Geometry: final body of the model. Coordinates: model frame, mm. A direction names the side the tool comes from. Coordinates: 2 decimals unless noted, no trailing zeros. Write each loop counter-clockwise with the first axis right and the second up, starting at its lowest first coordinate (ties: lowest second). Pieces come first, ordered by that corner, then holes.
from build123d import *

# Parameters (mm, degrees)
F0_W     = 150
F0_H     = 35
F1_DEPTH = 40
F2_D     = 5
F2_DEPTH = 50
F2_TIP   = 1.5021515476
F4_D     = 12
F4_DEPTH = 50
F4_TIP   = 3.6051637142
F5_D     = 20
F5_DEPTH = 50
F5_TIP   = 6.0086061903


with BuildPart() as f1:
    # F0 (on Top) → F1 (new body)
    with BuildSketch(Plane.XY):
        with Locations((0.152673311, -0.1323037595)):
            Rectangle(F0_W, F0_H)
    extrude(amount=F1_DEPTH)

    # F2
    with Locations(Plane(origin=(0, 0, 0), x_dir=(1, 0, 0), z_dir=(0, 0, -1))):
        with Locations((-59, -7.4576994487), (-69, 0.0423005513), (-59, 7.5423005513), (-49, 0.0423005513), (49, 0.0423005513), (59, -7.4576994487), (59, 7.5423005513), (69, 0.0423005513)):
            Hole(F2_D / 2, depth=F2_DEPTH)
            with Locations((0, 0, -(F2_DEPTH + F2_TIP / 2))):  # 118° drill point
                Cone(0, F2_D / 2, F2_TIP, mode=Mode.SUBTRACT)

    # F4
    with Locations(Plane.XZ.offset(17.6323037595)):
        with Locations((-7.847326689, 28.4498091787), (8.152673311, 28.4498091787), (-7.847326689, 12.4498091787), (8.152673311, 12.4498091787)):
            Hole(F4_D / 2, depth=F4_DEPTH)
            with Locations((0, 0, -(F4_DEPTH + F4_TIP / 2))):  # 118° drill point
                Cone(0, F4_D / 2, F4_TIP, mode=Mode.SUBTRACT)

    # F5
    with Locations(Plane.XZ.offset(17.6323037595)):
        with Locations((0.0776981695, 20)):
            Hole(F5_D / 2, depth=F5_DEPTH)
            with Locations((0, 0, -(F5_DEPTH + F5_TIP / 2))):  # 118° drill point
                Cone(0, F5_D / 2, F5_TIP, mode=Mode.SUBTRACT)


solid = f1.part
Item 1: Section D-D, the plane x = 7. Output: boundary loops of the cut face in (y, z), plus the area to 3 significant figures.
Derived:
outline: (-17.63, 0) - (17.37, 0) - (17.37, 6.56) - (-17.63, 6.56) - close; (-17.63, 34.34) - (17.37, 34.34) - (17.37, 40) - (-17.63, 40) - close
area: 428 mm2
Item 2: Section B-B, the plane z = 25. State how many separate pieces and enclosed holes the cut face has, plus the area to 3 significant figures.
Derived:
separate pieces: 2
enclosed holes: 8
area: 4,190 mm2
Item 3: Section C-C, the plane x = -59. Output: boundary loops of the cut face in (y, z), plus the area to 3 significant figures.
Derived:
outline: (-17.63, 0) - (-10.04, 0) - (-10.04, 40) - (-17.63, 40) - close; (-5.04, 0) - (4.96, 0) - (4.96, 40) - (-5.04, 40) - close; (9.96, 0) - (17.37, 0) - (17.37, 40) - (9.96, 40) - close
area: 1,000 mm2
Item 4: Set-up query: faces 4 (the cylindrical face through (-51.309, 0.915, 20.28)), 5 (the cylindrical face through (-9.914, 0.113, 20.398)). Return all of +Z, -Z, +X, -X, +Y, -Y with unobstructed straight access to the full face (end or side cutting, diameter ignored); none if empty.
Derived:
face 4: +Z, -Z
face 5: +Y, -Y
Item 5: Material intervals for probe 1 along Y at (x, z) = (-59, 17); probe 2 along Y at (x, z) = (-49, 21.5); probe 3 along X at (y, z) = (-9.5, 20), sorted ascending.
Derived:
probe 1: y = -17.63 to -10.04, -5.04 to 4.96, 9.96 to 17.37
probe 2: y = -17.63 to -2.54, 2.46 to 17.37
probe 3: x = -74.85 to -60.55, -57.45 to -9.92, 10.08 to 57.45, 60.55 to 75.15
Item 6: Section A-A, the plane x = 49. Output: boundary loops of the cut face in (y, z), plus the area to 3 significant figures.
Derived:
outline: (-17.63, 0) - (-2.54, 0) - (-2.54, 40) - (-17.63, 40) - close; (2.46, 0) - (17.37, 0) - (17.37, 40) - (2.46, 40) - close
area: 1,200 mm2
Item 7: Pull-direction query (Z, two-part tool) for faces 1 (the flat face through (-1, 0, 40)), 2 (the cylindrical face through (-71.385, -0.793, 20.28)), 3 (the cylindrical face through (0, 0, 30)); classes: released by +Z, released by -Z, zero draft, split by the parting line, or undercut.
Derived:
face 1: released by +Z
face 2: zero draft
face 3: undercut
Item 8: Pin query (flat end, axial travel): pin 1 (9.5 mm diameter, centred on x = 8.15, z = 12.45, fed in from -Y). Return the tip coordinate at first contact, or that it passes through.
Derived:
pin 1: passes through
